Read the model definition and answer for the solid it produces. Units are mm, in the model's axes. Face numbers are marked on the shaded views. A direction names the side the tool comes from. Give positions to 0.01 mm unless a question says otherwise; leave off trailing zeros. Order: outer loops, then holes, each group sorted by start corner. A loop starts at its lowest first (then second) coordinate and runs counter-clockwise, first axis right, second up. Notation, with made-up numbers: (12, 52.25) - (33, 52.25) arc R13 ccw to (33, 74.25) - close; hole circle Ø10 at (71.5, 86). An arc over 180 degrees is marked (long way). Return JSON: item names as keys, results as strings.
```python
from build123d import *

# Parameters (mm, degrees)
F0_R     = 10
F1_DEPTH = 40
F2_DEPTH = 24
F5_DEPTH = 10
F6_DEPTH = 30.001
F7_R     = 10


with BuildPart() as f1:
    # F0 (on Front) → F1 (new body, symmetric)
    with BuildSketch(Plane.XZ):
        Polygon((0, 30), (0, 0), (100, 0), (100, 30), (56, 30), align=None)
        with BuildLine():
            Line((56, 30), (100, 30))
            Line((100, 30), (100, 68))
            ThreePointArc((100, 68), (78, 90), (56, 68))
            Line((56, 68), (56, 30))
        make_face()
        with Locations((78, 68)):
            Circle(F0_R, mode=Mode.SUBTRACT)
    extrude(amount=F1_DEPTH, both=True)

    # F0 (on Front) → F2 (cut, symmetric)
    with BuildSketch(Plane.XZ):
        with BuildLine():
            Line((56, 30), (100, 30))
            Line((100, 30), (100, 68))
            ThreePointArc((100, 68), (78, 90), (56, 68))
            Line((56, 68), (56, 30))
        make_face()
        with Locations((78, 68)):
            Circle(F0_R, mode=Mode.SUBTRACT)
    extrude(amount=F2_DEPTH, both=True, mode=Mode.SUBTRACT)

    # F4 (on face) → F5 (cut)
    with BuildSketch(Plane.XY.offset(30)):
        with BuildLine():
            Line((0, -17), (24, -17))
            ThreePointArc((24, -17), (41, 0), (24, 17))
            Line((24, 17), (0, 17))
            Line((0, 17), (0, 9))
            Line((0, 9), (24, 9))
            ThreePointArc((24, 9), (33, 0), (24, -9))
            Line((24, -9), (0, -9))
            Line((0, -9), (0, -17))
        make_face()
        with BuildLine():
            Line((0, 9), (0, -9))
            Line((0, -9), (24, -9))
            ThreePointArc((24, -9), (33, 0), (24, 9))
            Line((24, 9), (0, 9))
        make_face()
    extrude(amount=-F5_DEPTH, mode=Mode.SUBTRACT)

    # F4 (on face) → F6 (cut, through all)
    with BuildSketch(Plane.XY.offset(30)):
        with BuildLine():
            Line((0, 9), (0, -9))
            Line((0, -9), (24, -9))
            ThreePointArc((24, -9), (33, 0), (24, 9))
            Line((24, 9), (0, 9))
        make_face()
    extrude(amount=-F6_DEPTH, mode=Mode.SUBTRACT)

    # F7
    f7_edges = [f1.edges().sort_by_distance(p)[0] for p in [
        (0, -40, 15),
        (0, 40, 15),
    ]]
    fillet(f7_edges, radius=F7_R)


solid = f1.part
```
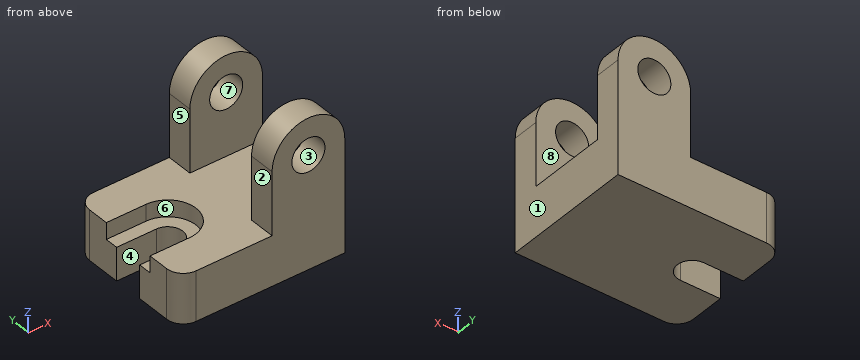
Q1. Consider L1, parallel to Z at x = 78, y = 30.75; L2, parallel to Y at x = 68.5, z = 50.5; L3, parallel to X at y = -34, z = 68.5. Determine where each line is inside the solid, lowest interval first.
Values:
{"L1": "z = 0 to 58, 78 to 90", "L2": "y = -40 to -24, 24 to 40", "L3": "x = 56.01 to 68.01, 87.99 to 99.99"}
Q2. For the marked faces 4, 5, 6, 7 and 8, determine the directions among +Z, -Z, +X, -X, +Y, -Y from which every point of the face is accessible in a straight line to the end or side of a thin tool.
Values:
{"face 4": "+Z, -Z, -X", "face 5": "+Z, -X, +Y, -Y", "face 6": "+Z, -X", "face 7": "+Y, -Y", "face 8": "+Z, +X, -X"}
Q3. Given pin 1 (8 mm diameter, centred on x = 60.5, y = 30.5, fed in from -Z); pin 2 (12 mm diameter, centred on x = 58, y = -1.5, fed in from +Z); pin 3 (18 mm diameter, centred on x = 78, z = 68, fed in from +Y); pin 4 (13 mm diameter, centred on y = -34, z = 57.5, fed in from -X), each flat-ended and moving along its own axis, determine where each tip first touches the part or whether it passes through.
Values:
{"pin 1": "stops at z = 0", "pin 2": "stops at z = 30", "pin 3": "passes through", "pin 4": "stops at x = 56"}
Q4. A cutting plane is placed at B-B (z = 39). Write down the section's boundary in (x, y), and give its area (3 significant figures).
Values:
{"outline": "(56, -40) - (100, -40) - (100, -24) - (56, -24) - close; (56, 24) - (100, 24) - (100, 40) - (56, 40) - close", "area": "1,410 mm²"}
Q5. A cutting plane is placed at C-C (z = 60). Write down the section's boundary in (x, y).
Values:
{"outline": "(56, -40) - (72, -40) - (72, -24) - (56, -24) - close; (56, 24) - (72, 24) - (72, 40) - (56, 40) - close; (84, -40) - (100, -40) - (100, -24) - (84, -24) - close; (84, 24) - (100, 24) - (100, 40) - (84, 40) - close"}
Q6. A cutting plane is placed at D-D (y = -33). Write down the section's boundary in (x, z), and give its area (3 significant figures).
Values:
{"outline": "(0.46, 0) - (100, 0) - (100, 68) arc R22 ccw to (56, 68) - (56, 30) - (0.46, 30) - close; hole circle Ø20 at (78, 68)", "area": "5,100 mm²"}
Q7. Determine the mould class of the marked faces 1, 2 and 3 for opening direction X: released by +X, released by -X, zero draft, split by the parting line, or undercut.
Values:
{"face 1": "released by +X", "face 2": "released by -X", "face 3": "undercut"}
Q8. A cutting plane is placed at A-A (x = 78). Write down the section's boundary in (y, z).
Values:
{"outline": "(-40, 0) - (40, 0) - (40, 58) - (24, 58) - (24, 30) - (-24, 30) - (-24, 58) - (-40, 58) - close; (-40, 78) - (-24, 78) - (-24, 90) - (-40, 90) - close; (24, 78) - (40, 78) - (40, 90) - (24, 90) - close"}
